Geometry: see drawing. Coordinates: mm, zero at the bounding-box minimum. A direction names the side the tool comes from. Give positions to 0.01 mm unless a question says otherwise; leave off trailing zeros. Loops run counter-clockwise (first coordinate to the right, second up) from the corner with the lowest first, then second, coordinate; pieces in that order, holes last. Notation, with made-up numbers: M 69.25,-22 L 128.25,-22 A8 ccw 128.25,-16 Z; hole C 70.5,81.25 d6. An arc over 180 degrees is marked long. Answer in a Markdown table with one row per item.
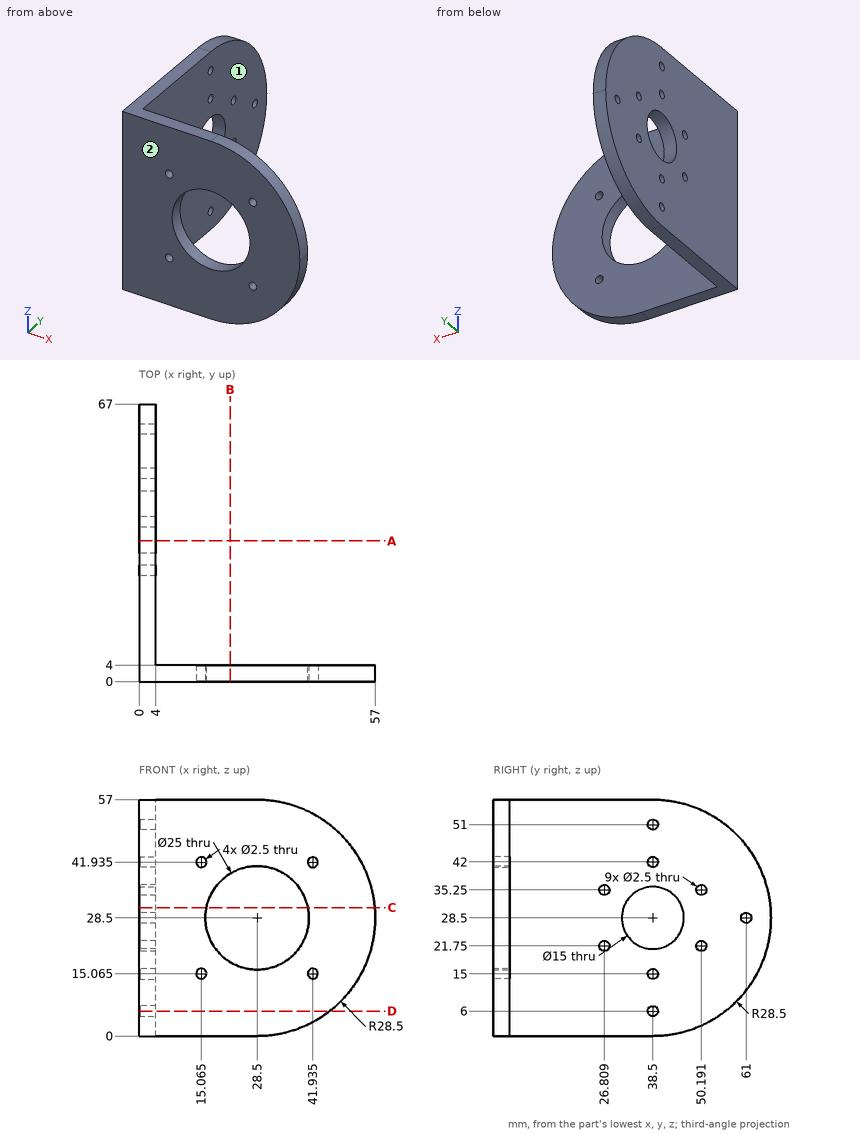
1) Set-up query: the marked faces 1 and 2. Return all of +Z, -Z, +X, -X, +Y, -Y with unobstructed straight access to the full face (end or side cutting, diameter ignored); none if empty.
Reply:
| item | result |
|---|---|
| face 1 | +Z, -Z, +X, +Y |
| face 2 | +Z, -Z, +X, -X, -Y |
2) Material intervals for L1, parallel to Z at x = 2, y = 38 (1 decimal); L2, parallel to X at y = 5.5, z = 33.5; L3, parallel to Y at x = 2.5, z = 35.25, sorted ascending.
Reply:
| item | result |
|---|---|
| L1 | z = 0 to 4.9, 7.1 to 13.9, 16.1 to 21, 36 to 40.9, 43.1 to 49.9, 52.1 to 57 |
| L2 | x = 0 to 4 |
| L3 | y = 0 to 25.56, 28.06 to 35.23, 41.77 to 48.94, 51.44 to 66.19 |
3) Section B-B, the plane x = 22. Return loops of the section in (y, z), then the cut area to 3 significant figures.
Reply:
| item | result |
|---|---|
| outline | M 0,0 L 4,0 L 4,17.82 L 0,17.82 Z; M 0,39.18 L 4,39.18 L 4,57 L 0,57 Z |
| area | 143 mm² |
4) Section A-A, the plane y = 34. Return loops of the section in (x, z).
Reply:
| item | result |
|---|---|
| outline | M 0,0 L 4,0 L 4,22.5 L 0,22.5 Z; M 0,34.5 L 4,34.5 L 4,57 L 0,57 Z |
5) Section C-C, the plane z = 31. Return loops of the section in (x, y).
Reply:
| item | result |
|---|---|
| outline | M 0,0 L 16.25,0 L 16.25,4 L 4,4 L 4,31.43 L 0,31.43 Z; M 0,45.57 L 4,45.57 L 4,66.89 L 0,66.89 Z; M 40.75,0 L 56.89,0 L 56.89,4 L 40.75,4 Z |
6) Pin query (flat end, axial travel): pin 1 Ø4 at (y, z) = (26.81, 21.75) entering from -X; pin 2 Ø3 at (y, z) = (50.19, 35.25) entering from +X; pin 3 Ø2 at (x, z) = (41.94, 15.06) entering from +Y. Return the tip coordinate at first contact, or that it passes through.
Reply:
| item | result |
|---|---|
| pin 1 | stops at x = 0 |
| pin 2 | stops at x = 4 |
| pin 3 | passes through |
7) Section D-D, the plane z = 6. Return loops of the section in (x, y).
Reply:
| item | result |
|---|---|
| outline | M 0,0 L 45.99,0 L 45.99,4 L 4,4 L 4,37.25 L 0,37.25 Z; M 0,39.75 L 4,39.75 L 4,55.99 L 0,55.99 Z |
